```python
from build123d import *

# Parameters (mm, degrees)
CROQUIS1_W                   = 80
CROQUIS1_H                   = 36
CROQUIS1_R                   = 2.125
CROQUIS1_R_2                 = 0.5
SALIENTE_EXTRUIR1_DEPTH      = 1.6
CROQUIS2_W                   = 70
CROQUIS2_H                   = 23
SALIENTE_EXTRUIR2_DEPTH      = 7
SALIENTE_EXTRUIR3_DEPTH      = 3
SALIENTE_EXTRUIR4_DEPTH      = 0.5
SALIENTE_EXTRUIR4_DEPTH_BACK = 9
CROQUIS6_R                   = 0.5
CORTAR_EXTRUIR1_DEPTH        = 0.1
REDONDEO1_R                  = 0.5
FILLET2_R                    = 0.1


with BuildPart() as part:
    # Croquis1 → Saliente-Extruir1 (new body)
    with BuildSketch(Plane.XY):
        with Locations((40, 18)):
            Rectangle(CROQUIS1_W, CROQUIS1_H)
        with Locations((2.5, 33.46)):
            Circle(CROQUIS1_R, mode=Mode.SUBTRACT)
        with Locations(Location((77.5, 33.51, 0), (0, 0, 180))):
            Circle(CROQUIS1_R, mode=Mode.SUBTRACT)
        with Locations((77.5, 2.49)):
            Circle(CROQUIS1_R, mode=Mode.SUBTRACT)
        with Locations(Location((2.5, 2.49, 0), (0, 0, 180))):
            Circle(CROQUIS1_R, mode=Mode.SUBTRACT)
        with Locations((8, 33.46)):
            Circle(CROQUIS1_R_2, mode=Mode.SUBTRACT)
        with Locations((10.53333, 33.46)):
            Circle(CROQUIS1_R_2, mode=Mode.SUBTRACT)
        with Locations((13.06666, 33.46)):
            Circle(CROQUIS1_R_2, mode=Mode.SUBTRACT)
        with Locations((15.59999, 33.46)):
            Circle(CROQUIS1_R_2, mode=Mode.SUBTRACT)
        with Locations((18.13332, 33.46)):
            Circle(CROQUIS1_R_2, mode=Mode.SUBTRACT)
        with Locations((20.66665, 33.46)):
            Circle(CROQUIS1_R_2, mode=Mode.SUBTRACT)
        with Locations((23.19998, 33.46)):
            Circle(CROQUIS1_R_2, mode=Mode.SUBTRACT)
        with Locations((25.73331, 33.46)):
            Circle(CROQUIS1_R_2, mode=Mode.SUBTRACT)
        with Locations((28.26664, 33.46)):
            Circle(CROQUIS1_R_2, mode=Mode.SUBTRACT)
        with Locations((30.79997, 33.46)):
            Circle(CROQUIS1_R_2, mode=Mode.SUBTRACT)
        with Locations((33.3333, 33.46)):
            Circle(CROQUIS1_R_2, mode=Mode.SUBTRACT)
        with Locations((35.86663, 33.46)):
            Circle(CROQUIS1_R_2, mode=Mode.SUBTRACT)
        with Locations((38.39996, 33.46)):
            Circle(CROQUIS1_R_2, mode=Mode.SUBTRACT)
        with Locations((40.93329, 33.46)):
            Circle(CROQUIS1_R_2, mode=Mode.SUBTRACT)
        with Locations((43.46662, 33.46)):
            Circle(CROQUIS1_R_2, mode=Mode.SUBTRACT)
        with Locations((45.99995, 33.46)):
            Circle(CROQUIS1_R_2, mode=Mode.SUBTRACT)
    extrude(amount=SALIENTE_EXTRUIR1_DEPTH)

    # Croquis2 → Saliente-Extruir2 (add)
    with BuildSketch(Plane.XY.offset(1.6)):
        with Locations((40, 18)):
            Rectangle(CROQUIS2_W, CROQUIS2_H)
    extrude(amount=SALIENTE_EXTRUIR2_DEPTH)

    # Croquis3 → Saliente-Extruir3 (add)
    with BuildSketch(Plane.XY.offset(1.6)):
        Polygon((79.437795719, 19.5), (75, 26.5), (75, 9.5), (79.437795719, 16.5), align=None)
    extrude(amount=SALIENTE_EXTRUIR3_DEPTH)

    # Croquis6 → Saliente-Extruir4 (add, two sides: drawn at the far end of the back side and taken through both)
    with BuildSketch(Plane.XY.offset(1.6).offset(-SALIENTE_EXTRUIR4_DEPTH_BACK)):
        with Locations((8, 33.46)):
            Circle(CROQUIS6_R)
        with Locations((10.53333, 33.46)):
            Circle(CROQUIS6_R)
        with Locations((13.06666, 33.46)):
            Circle(CROQUIS6_R)
        with Locations((15.59999, 33.46)):
            Circle(CROQUIS6_R)
        with Locations((18.13332, 33.46)):
            Circle(CROQUIS6_R)
        with Locations((20.66665, 33.46)):
            Circle(CROQUIS6_R)
        with Locations((23.19998, 33.46)):
            Circle(CROQUIS6_R)
        with Locations((25.73331, 33.46)):
            Circle(CROQUIS6_R)
        with Locations((28.26664, 33.46)):
            Circle(CROQUIS6_R)
        with Locations((30.79997, 33.46)):
            Circle(CROQUIS6_R)
        with Locations((33.3333, 33.46)):
            Circle(CROQUIS6_R)
        with Locations((35.86663, 33.46)):
            Circle(CROQUIS6_R)
        with Locations((38.39996, 33.46)):
            Circle(CROQUIS6_R)
        with Locations((40.93329, 33.46)):
            Circle(CROQUIS6_R)
        with Locations((43.46662, 33.46)):
            Circle(CROQUIS6_R)
        with Locations((45.99995, 33.46)):
            Circle(CROQUIS6_R)
    extrude(amount=SALIENTE_EXTRUIR4_DEPTH + SALIENTE_EXTRUIR4_DEPTH_BACK)

    # Croquis7 → Cortar-Extruir1 (cut)
    with BuildSketch(Plane.XY.offset(8.6)):
        with BuildLine():
            Line((8.25, 24.9), (71.75, 24.9))
            ThreePointArc((71.75, 24.9), (72.103553391, 24.753553391), (72.25, 24.4))
            Line((72.25, 24.4), (72.25, 11.6))
            ThreePointArc((72.25, 11.6), (72.103553391, 11.246446609), (71.75, 11.1))
            Line((71.75, 11.1), (8.25, 11.1))
            ThreePointArc((8.25, 11.1), (7.896446609, 11.246446609), (7.75, 11.6))
            Line((7.75, 11.6), (7.75, 24.4))
            ThreePointArc((7.75, 24.4), (7.896446609, 24.753553391), (8.25, 24.9))
        make_face()
    extrude(amount=-CORTAR_EXTRUIR1_DEPTH, mode=Mode.SUBTRACT)

    # Redondeo1
    redondeo1_edges = [part.edges().sort_by_distance(p)[0] for p in [
        (5, 6.5, 5.1),
        (75, 6.5, 5.1),
        (75, 29.5, 5.1),
        (5, 29.5, 5.1),
    ]]
    fillet(redondeo1_edges, radius=REDONDEO1_R)

    # Fillet2
    fillet2_edges = [part.edges().sort_by_distance(p)[0] for p in [
        (40, 6.5, 8.6),
        (5, 18, 8.6),
        (75, 18, 8.6),
        (40, 29.5, 8.6),
        (74.853553391, 6.646446609, 8.6),
        (74.853553391, 29.353553391, 8.6),
        (5.146446609, 29.353553391, 8.6),
        (5.146446609, 6.646446609, 8.6),
    ]]
    fillet(fillet2_edges, radius=FILLET2_R)


solid = part.part
```
Design review of the part built by this model. Coordinates are the model's own, in mm. A direction names the side the tool comes from. Give positions to 0.01 mm unless a question says otherwise; leave off trailing zeros. Loops run counter-clockwise (first coordinate to the right, second up) from the corner with the lowest first, then second, coordinate; pieces in that order, holes last. Notation, with made-up numbers: (-24.75, 75.5) -> (-9.75, 75.5) arc R15 ccw to (-9.75, 91.5) -> close; hole circle Ø8 at (26.5, -25). An arc over 180 degrees is marked (long way). One line per item, written item: value.
Q1. We need section C-C on x = 59. Give the boundary of the cut face in (y, z).
Numbers:
outline: (0, 0) -> (36, 0) -> (36, 1.6) -> (29.5, 1.6) -> (29.5, 8.5) arc R0.1 ccw to (29.4, 8.6) -> (24.9, 8.6) -> (24.9, 8.5) -> (11.1, 8.5) -> (11.1, 8.6) -> (6.6, 8.6) arc R0.1 ccw to (6.5, 8.5) -> (6.5, 1.6) -> (0, 1.6) -> close
Q2. Machinability: for faces 4 (the flat face through (5, 18, 5)), 5 (the flat face through (40, 18, 8.5)), 6 (the flat face through (79.438, 18, 3)), which of the approach directions +Z, -Z, +X, -X, +Y, -Y give a long, thin tool a straight path to every point of the face, cutting with its end or side? Answer none if there is none.
Numbers:
face 4: +Z, -X, +Y, -Y
face 5: +Z
face 6: +Z, +X, +Y, -Y
Q3. For pin 1 Ø4 at (x, y) = (55, 16) entering from +Z; pin 2 Ø1.5 at (x, y) = (51, 32) entering from -Z; pin 3 Ø0.8 at (x, y) = (31, 33.5) entering from +Z, all flat-tipped, find the tip position at first contact; note any pin that passes through.
Numbers:
pin 1: stops at z = 8.5
pin 2: stops at z = 0
pin 3: stops at z = 2.1
Q4. We need section D-D on z = 5.75. Give the boundary of the cut face in (x, y).
Numbers:
outline: (5, 7) arc R0.5 ccw to (5.5, 6.5) -> (74.5, 6.5) arc R0.5 ccw to (75, 7) -> (75, 29) arc R0.5 ccw to (74.5, 29.5) -> (5.5, 29.5) arc R0.5 ccw to (5, 29) -> close
Q5. We need section A-A on z = -2.5. Give the number of separate pieces and of enclosed holes in the cut face, and give its area (3 significant figures).
Numbers:
separate pieces: 16
enclosed holes: 0
area: 12.6 mm^2
Q6. We need section B-B on x = 2.5. Give the boundary of the cut face in (y, z) (3 decimals), and give its area (3 significant figures).
Numbers:
outline: (0, 0) -> (0.365, 0) -> (0.365, 1.6) -> (0, 1.6) -> close; (4.615, 0) -> (31.335, 0) -> (31.335, 1.6) -> (4.615, 1.6) -> close; (35.585, 0) -> (36, 0) -> (36, 1.6) -> (35.585, 1.6) -> close
area: 44.0 mm^2
Q7. For L1, parallel to Y at x = 77.5, z = 1.2 (3 decimals); L2, parallel to X at y = 33.51, z = 0.7 (3 decimals); L3, parallel to Y at x = 2.5, z = 0.95 (3 decimals), list the stretches that pass through material, from the lowest coordinate up.
Numbers:
L1: y = 0 to 0.365, 4.615 to 31.385, 35.635 to 36
L2: x = 0 to 0.376, 4.624 to 75.375, 79.625 to 80
L3: y = 0 to 0.365, 4.615 to 31.335, 35.585 to 36
Q8. Draft analysis for pull direction Y (two halves, no side actions). For faces 1 (the flat face through (77.25, 22.95, 3.08)), 2 (the flat face through (77, 18, 4.6)), 3 (the cylindrical face through (79.19, 34.8, 0.79)), state which applies: pulls with the +Y half, pulls with the -Y half, needs draft (parallel to the pull), parting line crosses it, or undercut.
Numbers:
face 1: pulls with the +Y half
face 2: needs draft
face 3: undercut
